from build123d import *

# Parameters (mm, degrees)
RESSALTO_EXTRUS_O1_DEPTH = 1000
ESBO_O4_R                = 3.5
CORTE_EXTRUS_O1_DEPTH    = 22.900000388
ESBO_O5_R                = 5.5
CORTE_EXTRUS_O2_DEPTH    = 8.9


with BuildPart() as part:
    # Esboço2 → Ressalto-extrusão1 (new body)
    with BuildSketch(Plane.XY):
        with BuildLine():
            Line((-1.14927176, 21.393056679), (-1.14927176, 1.393056679))
            Line((-1.14927176, 1.393056679), (0.35072824, -0.106943321))
            Line((0.35072824, -0.106943321), (4.94937774, -0.106943321))
            Line((4.94937774, -0.106943321), (8.749377483, 3.693056422))
            Line((8.749377483, 3.693056422), (12.130866629, 3.693056422))
            Line((12.130866629, 3.693056422), (13.36057142, 2.463351631))
            ThreePointArc((13.36057142, 2.463351631), (14.896988246, 1.734969723), (15.625370154, 0.198552898))
            Line((15.625370154, 0.198552898), (15.830866097, -0.006942978))
            Line((15.830866097, -0.006942978), (17.859427097, -0.006942978))
            Line((17.859427097, -0.006942978), (18.077094898, 0.210724894))
            ThreePointArc((18.077094898, 0.210724894), (18.804225931, 1.734970575), (20.328471586, 2.462101662))
            Line((20.328471586, 2.462101662), (20.750728628, 2.884358639))
            Line((20.750728628, 2.884358639), (20.750728628, 19.901756343))
            Line((20.750728628, 19.901756343), (20.328471651, 20.324013385))
            ThreePointArc((20.328471651, 20.324013385), (18.804226447, 21.0511438), (18.077094898, 22.575388463))
            Line((18.077094898, 22.575388463), (17.859427097, 22.793056335))
            Line((17.859427097, 22.793056335), (15.830866097, 22.793056335))
            Line((15.830866097, 22.793056335), (15.625370154, 22.58756046))
            ThreePointArc((15.625370154, 22.58756046), (14.896988246, 21.051143635), (13.36057142, 20.322761727))
            Line((13.36057142, 20.322761727), (12.130866629, 19.093056935))
            Line((12.130866629, 19.093056935), (8.749377483, 19.093056935))
            Line((8.749377483, 19.093056935), (4.94937774, 22.893056679))
            Line((4.94937774, 22.893056679), (0.35072824, 22.893056679))
            Line((0.35072824, 22.893056679), (-1.14927176, 21.393056679))
        make_face()
    extrude(amount=RESSALTO_EXTRUS_O1_DEPTH)

    # Esboço4 → Corte-extrusão1 (cut, through all)
    with BuildSketch(Plane(origin=(20.750728628, 0, 0), x_dir=(0, 0, -1), z_dir=(1, 0, 0))):
        with Locations((-50, 11.393057491)):
            Circle(ESBO_O4_R)
        with Locations((-110, 11.393057491)):
            Circle(ESBO_O4_R)
        with Locations((-170, 11.393057491)):
            Circle(ESBO_O4_R)
        with Locations((-230, 11.393057491)):
            Circle(ESBO_O4_R)
        with Locations((-290, 11.393057491)):
            Circle(ESBO_O4_R)
        with Locations((-350, 11.393057491)):
            Circle(ESBO_O4_R)
        with Locations((-410, 11.393057491)):
            Circle(ESBO_O4_R)
        with Locations((-470, 11.393057491)):
            Circle(ESBO_O4_R)
        with Locations((-530, 11.393057491)):
            Circle(ESBO_O4_R)
        with Locations((-590, 11.393057491)):
            Circle(ESBO_O4_R)
        with Locations((-650, 11.393057491)):
            Circle(ESBO_O4_R)
        with Locations((-710, 11.393057491)):
            Circle(ESBO_O4_R)
        with Locations((-770, 11.393057491)):
            Circle(ESBO_O4_R)
        with Locations((-830, 11.393057491)):
            Circle(ESBO_O4_R)
        with Locations((-890, 11.393057491)):
            Circle(ESBO_O4_R)
        with Locations((-950, 11.393057491)):
            Circle(ESBO_O4_R)
    extrude(amount=-CORTE_EXTRUS_O1_DEPTH, mode=Mode.SUBTRACT)

    # Esboço5 → Corte-extrusão2 (cut)
    with BuildSketch(Plane(origin=(20.750728628, 0, 0), x_dir=(0, 0, -1), z_dir=(1, 0, 0))):
        with Locations((-50, 11.393057491)):
            Circle(ESBO_O5_R)
        with Locations((-110, 11.393057491)):
            Circle(ESBO_O5_R)
        with Locations((-170, 11.393057491)):
            Circle(ESBO_O5_R)
        with Locations((-230, 11.393057491)):
            Circle(ESBO_O5_R)
        with Locations((-290, 11.393057491)):
            Circle(ESBO_O5_R)
        with Locations((-350, 11.393057491)):
            Circle(ESBO_O5_R)
        with Locations((-410, 11.393057491)):
            Circle(ESBO_O5_R)
        with Locations((-470, 11.393057491)):
            Circle(ESBO_O5_R)
        with Locations((-530, 11.393057491)):
            Circle(ESBO_O5_R)
        with Locations((-590, 11.393057491)):
            Circle(ESBO_O5_R)
        with Locations((-650, 11.393057491)):
            Circle(ESBO_O5_R)
        with Locations((-710, 11.393057491)):
            Circle(ESBO_O5_R)
        with Locations((-770, 11.393057491)):
            Circle(ESBO_O5_R)
        with Locations((-830, 11.393057491)):
            Circle(ESBO_O5_R)
        with Locations((-890, 11.393057491)):
            Circle(ESBO_O5_R)
        with Locations((-950, 11.393057491)):
            Circle(ESBO_O5_R)
    extrude(amount=-CORTE_EXTRUS_O2_DEPTH, mode=Mode.SUBTRACT)


solid = part.part
The model under review builds one solid part; all positions refer to its coordinate system, in mm. Round coordinates to 2 decimals unless told otherwise and drop trailing zeros. Write each loop counter-clockwise with the first axis right and the second up, starting at its lowest first coordinate (ties: lowest second). Pieces come first, ordered by that corner, then holes. Notation, with made-up numbers: M 8,-39.5 L 48,-39.5 A10 ccw 48,-21.5 Z; hole C 42.5,35 d2. An arc over 180 degrees is marked long. Use a Markdown table: item, result. Add a question column.
Q1. Insertion check: pin 1 (3.5 mm diameter, centred on y = 10, z = 530, fed in from +X); pin 2 (3.5 mm diameter, centred on y = 10, z = 587.5, fed in from +X). Each pin has a flat end and moves straight along its axis. Give the tip position at first contact, or say it passes through.
Q2. We need section A-A, the plane z = 800. State the section outline as (x, y) points.
Q3. To check wall thickness, follow line 1 (Y direction, x = 9, z = 290); line 2 (Y direction, x = 4.5, z = 170); line 3 (Y direction, x = 10.75, z = 630.5). State the ranges of each line that lie inside material, in increasing order.
Findings below:
| question | item | result |
|---|---|---|
| 1 | pin 1 | passes through |
| 1 | pin 2 | stops at x = 11.85 |
| 2 | outline | M -1.15,1.39 L 0.35,-0.11 L 4.95,-0.11 L 8.75,3.69 L 12.13,3.69 L 13.36,2.46 A2.53 cw 15.63,0.2 L 15.83,-0.01 L 17.86,-0.01 L 18.08,0.21 A2.53 cw 20.33,2.46 L 20.75,2.88 L 20.75,19.9 L 20.33,20.32 A2.53 cw 18.08,22.58 L 17.86,22.79 L 15.83,22.79 L 15.63,22.59 A2.53 cw 13.36,20.32 L 12.13,19.09 L 8.75,19.09 L 4.95,22.89 L 0.35,22.89 L -1.15,21.39 Z |
| 3 | line 1 | y = 3.69 to 7.89, 14.89 to 19.09 |
| 3 | line 2 | y = -0.11 to 7.89, 14.89 to 22.89 |
| 3 | line 3 | y = 3.69 to 19.09 |
